For this review, use the dimensioned drawing (mm, ordinates from the lowest corner) and the shaded views. A direction names the side the tool comes from. Round coordinates to 2 decimals unless told otherwise and drop trailing zeros. Order: outer loops, then holes, each group sorted by start corner. A loop starts at its lowest first (then second) coordinate and runs counter-clockwise, first axis right, second up. Notation, with made-up numbers: M 53,-14.75 L 66,-14.75 A13 cw 66,3.25 Z; hole C 57,49.5 d10. An arc over 180 degrees is marked long. One line per item, written item: value. Start each with the question number.
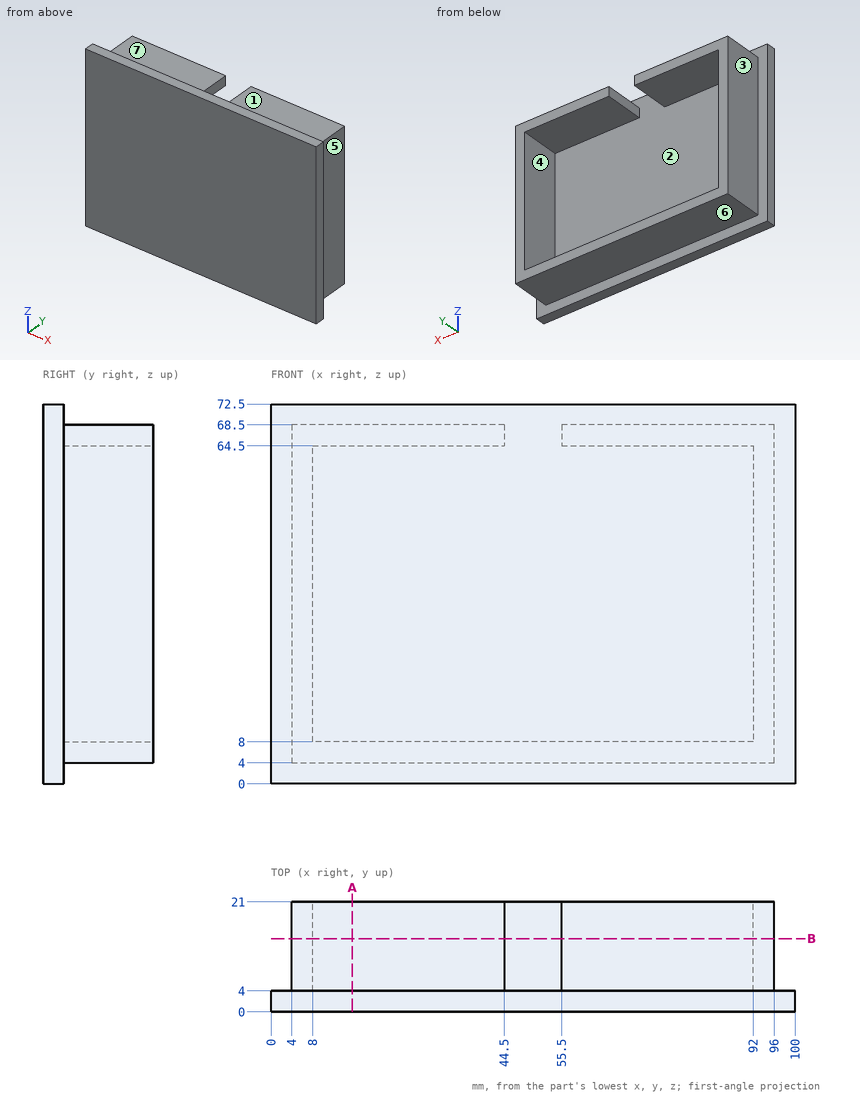
Item 1: Consider section B-B, the plane y = 14. Give the boundary of the cut face in (x, z), then the cut area to 3 significant figures.
Item 2: Machinability: for the marked faces 4, 5, 6 and 7, which of the approach directions +Z, -Z, +X, -X, +Y, -Y give a long, thin tool a straight path to every point of the face, cutting with its end or side? Answer none if there is none.
Item 3: Consider section A-A, the plane x = 15.5. Give the boundary of the cut face in (y, z).
Item 4: The part is to be moulded in two halves that separate along Z. For the marked faces 1, 2 and 3, say which applies: pulls with the +Z half, pulls with the -Z half, needs draft (parallel to the pull), parting line crosses it, or undercut.
Item 5: Clearance check with flat-ended pins moving along their axes: P1, Ø3, axis at x = 78.5, z = 40.5, coming from the +Y side; P2, Ø8.5, axis at x = 41.5, y = 11.5, coming from the -Z side; P3, Ø1.2, axis at y = 10, z = 65.5, coming from the -X side. State where each tip first meets the part, or that it passes through.
Item 6: Wall thickness on L1, parallel to X at y = 11, z = 9; L2, parallel to Z at x = 77.5, y = 13.5; L3, parallel to X at y = 19, z = 67: over which ranges is each line inside the solid? List them lowest first.
Computed:
1. outline: M 4,4 L 96,4 L 96,68.5 L 55.5,68.5 L 55.5,64.5 L 92,64.5 L 92,8 L 8,8 L 8,64.5 L 44.5,64.5 L 44.5,68.5 L 4,68.5 Z
1. area: 1,140 mm^2
2. face 4: +Y
2. face 5: +Z, -Z, +X, +Y
2. face 6: -Z, +X, -X, +Y
2. face 7: +Z, +X, -X, +Y
3. outline: M 0,0 L 4,0 L 4,4 L 21,4 L 21,8 L 4,8 L 4,64.5 L 21,64.5 L 21,68.5 L 4,68.5 L 4,72.5 L 0,72.5 Z
4. face 1: pulls with the +Z half
4. face 2: undercut
4. face 3: needs draft
5. P1: stops at y = 4
5. P2: stops at z = 4
5. P3: stops at x = 4
6. L1: x = 4 to 8, 92 to 96
6. L2: z = 4 to 8, 64.5 to 68.5
6. L3: x = 4 to 44.5, 55.5 to 96
